The drawing under review shows one solid part. Ordinate dimensions are in mm from its lowest x, y, z. A direction names the side the tool comes from. Coordinates: 2 decimals unless noted, no trailing zeros. Loops run counter-clockwise (first coordinate to the right, second up) from the corner with the lowest first, then second, coordinate; pieces in that order, holes last. Notation, with made-up numbers: M 23,32.5 L 58,32.5 A17 cw 58,57.5 Z; hole C 22,57.25 d4. An arc over 180 degrees is marked long. Put each result on its own line as item: value.
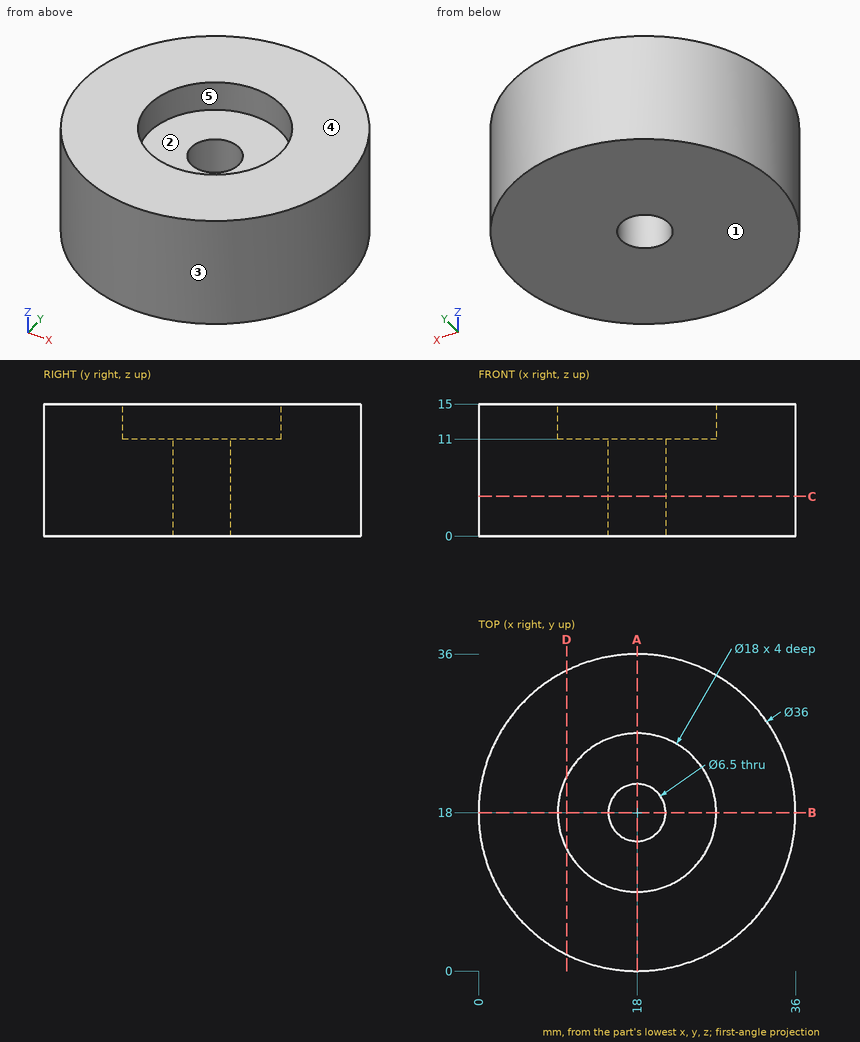
(1) Add section A-A (x = 18). Write out the cut boundary in (y, z), plus the area to 4 significant figures.
Determined:
outline: M 0,0 L 14.75,0 L 14.75,11 L 9,11 L 9,15 L 0,15 Z; M 21.25,0 L 36,0 L 36,15 L 27,15 L 27,11 L 21.25,11 Z
area: 396.5 mm^2
(2) Wall thickness on line 1 along Y through (x, z) = (18, 3.5); line 2 along Y through (x, z) = (16.5, 11.25); line 3 along Z through (x, y) = (16, 23.5): over which ranges is each line inside the solid? List them lowest first. Write a range as [from, to].
Determined:
line 1: y = [0, 14.75], [21.25, 36]
line 2: y = [0.06, 9.13], [26.87, 35.94]
line 3: z = [0, 11]
(3) For pin 1 (3 mm diameter, centred on x = 18.5, z = 9.5, fed in from +Y); pin 2 (4 mm diameter, centred on x = 9.5, z = 5, fed in from +Y); pin 3 (16 mm diameter, centred on x = 18, y = 18, fed in from +Z), all flat-tipped, find the tip position at first contact; note any pin that passes through.
Determined:
pin 1: stops at y = 36
pin 2: stops at y = 34.79
pin 3: stops at z = 11
(4) Draft analysis for pull direction X (two halves, no side actions). For the marked faces 3, 4 and 5, state which applies: +X half, -X half, draft (parallel to the pull), parting line (faces both ways), or undercut.
Determined:
face 3: parting line
face 4: draft
face 5: undercut
(5) Tool access review of the marked faces 1 and 2: name each direction out of +Z, -Z, +X, -X, +Y, -Y from which nothing blocks a thin tool from reaching the whole face with its end or side.
Determined:
face 1: -Z, +X, -X, +Y, -Y
face 2: +Z
(6) Add section D-D (x = 10). Write out the cut boundary in (y, z), plus the area to 3 significant figures.
Determined:
outline: M 1.88,0 L 34.12,0 L 34.12,15 L 22.12,15 L 22.12,11 L 13.88,11 L 13.88,15 L 1.88,15 Z
area: 451 mm^2
(7) Add section C-C (z = 4.5). Write out the cut boundary in (x, y), plus the area to 3 significant figures.
Determined:
outline: C 18,18 d36; hole C 18,18 d6.5
area: 985 mm^2
